Verification items for the finished model (mm, model axes). Round coordinates to 2 decimals unless told otherwise and drop trailing zeros. Order: outer loops, then holes, each group sorted by start corner. A loop starts at its lowest first (then second) coordinate and runs counter-clockwise, first axis right, second up. Notation, with made-up numbers: (51, 85) -> (103, 85) arc R21 cw to (103, 115) -> close; hole circle Ø10 at (73.5, 14). An arc over 180 degrees is marked (long way). Put each result on its own line as item: value.
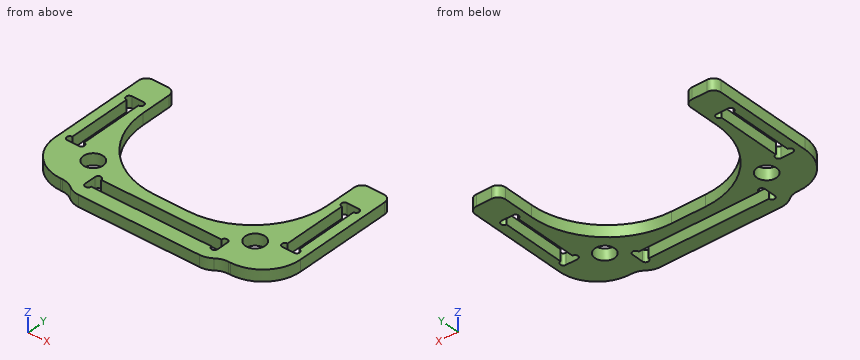
```python
from build123d import *

# Parameters (mm, degrees)
BOSS_EXTRUDE1_DEPTH = 3
FILLET1_R           = 20
CUT_EXTRUDE1_DEPTH  = 51.092414595
SKETCH3_R           = 2.6
CUT_EXTRUDE2_DEPTH  = 51.092414595
FILLET2_R           = 10
FILLET3_R           = 2
SKETCH4_W           = 36
SKETCH4_H           = 2
BOSS_EXTRUDE2_DEPTH = 3
FILLET4_R           = 5
FILLET5_R           = 5


with BuildPart() as part:
    # Sketch1 → Boss-Extrude1 (new body)
    with BuildSketch(Plane.XY):
        Polygon((0, 0), (-32.5, 0), (-32.5, 38), (-24.5, 38), (-24.5, 8), (0, 8), (24.5, 8), (24.5, 38), (32.5, 38), (32.5, 0), align=None)
    extrude(amount=BOSS_EXTRUDE1_DEPTH)

    # Fillet1
    fillet1_edges = [part.edges().sort_by_distance(p)[0] for p in [
        (24.5, 8, 1.5),
        (-24.5, 8, 1.5),
    ]]
    fillet(fillet1_edges, radius=FILLET1_R)

    # Sketch2 → Cut-Extrude1 (cut, through all)
    with BuildSketch(Plane.XY.offset(3)):
        with BuildLine():
            Line((-30, 10.9), (-26.9, 10.9))
            ThreePointArc((-26.9, 10.9), (-26.1, 11.7), (-26.9, 12.5))
            Line((-26.9, 12.5), (-26.9, 29.3))
            ThreePointArc((-26.9, 29.3), (-26.1, 30.1), (-26.9, 30.9))
            Line((-26.9, 30.9), (-30, 30.9))
            ThreePointArc((-30, 30.9), (-30.8, 30.1), (-30, 29.3))
            Line((-30, 29.3), (-30, 12.5))
            ThreePointArc((-30, 12.5), (-30.8, 11.7), (-30, 10.9))
        make_face()
        with BuildLine():
            Line((26.9, 12.5), (26.9, 29.3))
            ThreePointArc((26.9, 29.3), (26.1, 30.1), (26.9, 30.9))
            Line((26.9, 30.9), (30, 30.9))
            ThreePointArc((30, 30.9), (30.8, 30.1), (30, 29.3))
            Line((30, 29.3), (30, 12.5))
            ThreePointArc((30, 12.5), (30.8, 11.7), (30, 10.9))
            Line((30, 10.9), (26.9, 10.9))
            ThreePointArc((26.9, 10.9), (26.1, 11.7), (26.9, 12.5))
        make_face()
        with BuildLine():
            Line((-15.9, 1.81), (15.9, 1.81))
            ThreePointArc((15.9, 1.81), (16.7, 1.01), (17.5, 1.81))
            Line((17.5, 1.81), (17.5, 4.91))
            ThreePointArc((17.5, 4.91), (16.7, 5.71), (15.9, 4.91))
            Line((15.9, 4.91), (-15.9, 4.91))
            ThreePointArc((-15.9, 4.91), (-16.7, 5.71), (-17.5, 4.91))
            Line((-17.5, 4.91), (-17.5, 1.81))
            ThreePointArc((-17.5, 1.81), (-16.7, 1.01), (-15.9, 1.81))
        make_face()
    extrude(amount=-CUT_EXTRUDE1_DEPTH, mode=Mode.SUBTRACT)

    # Sketch3 → Cut-Extrude2 (cut, through all)
    with BuildSketch(Plane.XY.offset(3)):
        with Locations((-21.4, 8.91)):
            Circle(SKETCH3_R)
        with Locations(Location((21.4, 8.91, 0), (0, 0, 180))):
            Circle(SKETCH3_R)
    extrude(amount=-CUT_EXTRUDE2_DEPTH, mode=Mode.SUBTRACT)

    # Fillet2
    fillet2_edges = [part.edges().sort_by_distance(p)[0] for p in [
        (32.5, 0, 1.5),
        (-32.5, 0, 1.5),
    ]]
    fillet(fillet2_edges, radius=FILLET2_R)

    # Fillet3
    fillet3_edges = [part.edges().sort_by_distance(p)[0] for p in [
        (24.5, 38, 1.5),
        (32.5, 38, 1.5),
        (-32.5, 38, 1.5),
        (-24.5, 38, 1.5),
    ]]
    fillet(fillet3_edges, radius=FILLET3_R)

    # Sketch4 → Boss-Extrude2 (add)
    with BuildSketch(Plane.XY.offset(3)):
        with Locations((0, -1)):
            Rectangle(SKETCH4_W, SKETCH4_H)
    extrude(amount=-BOSS_EXTRUDE2_DEPTH)

    # Fillet4
    # the kernel refuses this fillet: 5 mm, written as the material it adds along each edge
    with BuildSketch(Plane(origin=(-18, 0, 3), x_dir=(-1, 0, 0), z_dir=(0, 0, -1))) as fillet4_piece_1:
        with BuildLine():
            CenterArc((4, -5), FILLET4_R, 90, 53.130102354)
            Line((0, -2), (0, 0))
            Line((0, 0), (4, 0))
        make_face()
    extrude(amount=3)
    with BuildSketch(Plane(origin=(18, 0, 3), x_dir=(1, 0, 0), z_dir=(0, 0, -1))) as fillet4_piece_2:
        with BuildLine():
            CenterArc((4, 5), FILLET4_R, 216.869897646, 53.130102354)
            Line((0, 2), (0, 0))
            Line((0, 0), (4, 0))
        make_face()
    extrude(amount=3)

    # Fillet5
    fillet5_edges = [part.edges().sort_by_distance(p)[0] for p in [
        (-18, -2, 1.5),
        (18, -2, 1.5),
    ]]
    fillet(fillet5_edges, radius=FILLET5_R)


solid = part.part
```
Item 1: Depth check by flat-ended pin: pin 1 Ø0.9 at (x, z) = (-1.5, 2) entering from +Y; pin 2 Ø1 at (x, z) = (7, 2.5) entering from +Y. Enter the tip coordinate at first touch or a pass-through.
Geometry check:
pin 1: y = 8
pin 2: y = 8.23
Item 2: Material ranges on line 1 along X through (y, z) = (33.5, 2.5); line 2 along X through (y, z) = (27.5, 2.5); line 3 along X through (y, z) = (12, 1.7), recorded low to high.
Geometry check:
line 1: -32.5 to -24.5, 24.5 to 32.5
line 2: -32.5 to -30, -26.9 to -24.49, 24.49 to 26.9, 30 to 32.5
line 3: -32.5 to -30.74, -26.16 to -16.5, 16.5 to 26.16, 30.74 to 32.5
Item 3: Sectioned sample at B-B, the plane y = 30.1. Record the boundary of the cut face in (x, z).
Geometry check:
outline: (-32.5, 0) -> (-30.8, 0) -> (-30.8, 3) -> (-32.5, 3) -> close; (-26.1, 0) -> (-24.5, 0) -> (-24.5, 3) -> (-26.1, 3) -> close; (24.5, 0) -> (26.1, 0) -> (26.1, 3) -> (24.5, 3) -> close; (30.8, 0) -> (32.5, 0) -> (32.5, 3) -> (30.8, 3) -> close
Item 4: Sectioned sample at D-D, the plane x = 9. Record the boundary of the cut face in (y, z), then the cut area to 3 significant figures.
Geometry check:
outline: (-2, 0) -> (1.81, 0) -> (1.81, 3) -> (-2, 3) -> close; (4.91, 0) -> (8.51, 0) -> (8.51, 3) -> (4.91, 3) -> close
area: 22.2 mm2
Item 5: Sectioned sample at A-A, the plane x = 0. Record the boundary of the cut face in (y, z), then the cut area to 3 significant figures.
Geometry check:
outline: (-2, 0) -> (1.81, 0) -> (1.81, 3) -> (-2, 3) -> close; (4.91, 0) -> (8, 0) -> (8, 3) -> (4.91, 3) -> close
area: 20.7 mm2
Item 6: Sectioned sample at C-C, the plane z = 0.85. Give the number of separate pieces and of enclosed holes in the cut face, then the cut area to 3 significant figures.
Geometry check:
separate pieces: 1
enclosed holes: 5
area: 914 mm2
